Source: three-view drawing plus pictorial views. Frame: mm from the lowest corner of the part. Round coordinates to 2 decimals unless told otherwise and drop trailing zeros. Order: outer loops, then holes, each group sorted by start corner. A loop starts at its lowest first (then second) coordinate and runs counter-clockwise, first axis right, second up. Notation, with made-up numbers: (-7, -29.75) -> (49, -29.75) arc R24 ccw to (49, -12.75) -> close; hole circle Ø9 at (72.25, -31.5). An arc over 180 degrees is marked (long way). Use a Markdown table: item, result.
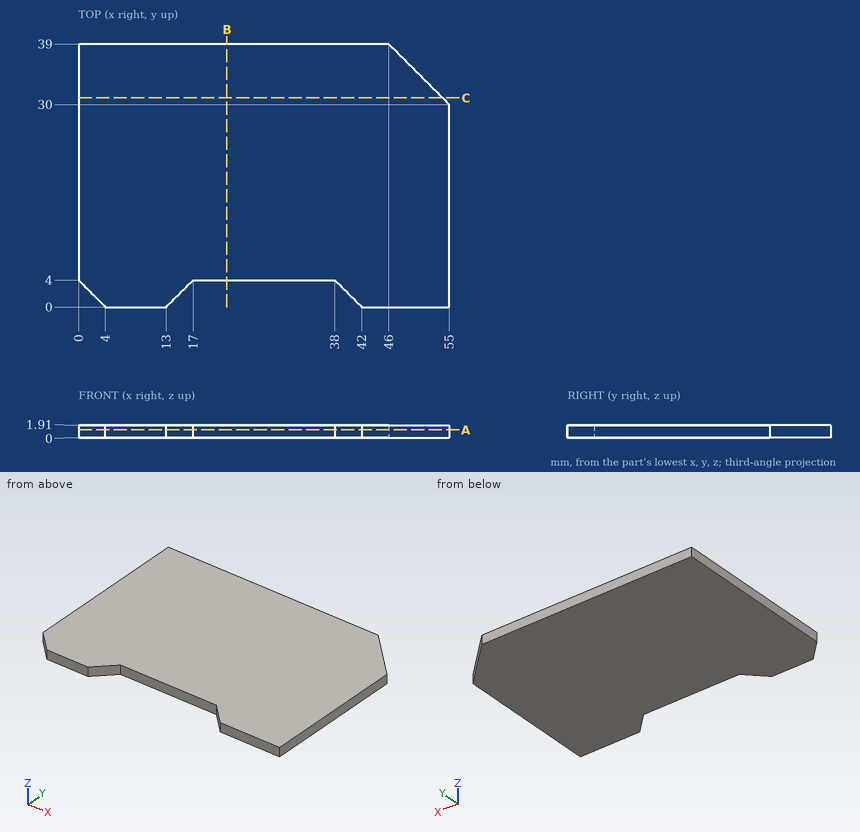
1) Cut plane C-C on y = 31. Return loops of the section in (x, z), and give its area (3 significant figures).
Results found:
| item | result |
|---|---|
| outline | (0, 0) -> (54, 0) -> (54, 1.91) -> (0, 1.91) -> close |
| area | 103 mm² |
2) Line query: L1, parallel to Y at x = 34.5, z = 1; L2, parallel to X at y = 2.5, z = 0.4; L3, parallel to X at y = 37, z = 1.1. Output: solid intervals per line, ascending. Write a range as [from, to].
Results found:
| item | result |
|---|---|
| L1 | y = [4, 39] |
| L2 | x = [1.5, 15.5], [39.5, 55] |
| L3 | x = [0, 48] |
3) Cut plane B-B on x = 22. Return loops of the section in (y, z), and give its area (4 significant figures).
Results found:
| item | result |
|---|---|
| outline | (4, 0) -> (39, 0) -> (39, 1.91) -> (4, 1.91) -> close |
| area | 66.85 mm² |
4) Cut plane A-A on z = 1.2. Return loops of the section in (x, y), and give its area (3 significant figures).
Results found:
| item | result |
|---|---|
| outline | (0, 4) -> (4, 0) -> (13, 0) -> (17, 4) -> (38, 4) -> (42, 0) -> (55, 0) -> (55, 30) -> (46, 39) -> (0, 39) -> close |
| area | 2,000 mm² |
